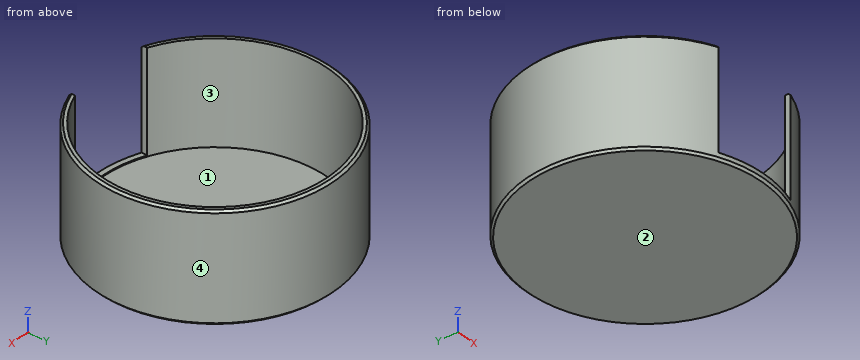
```python
from build123d import *

# Parameters (mm, degrees)
F0_R     = 55.5
F1_DEPTH = 50
F2_T     = -2.5
F4_DEPTH = 47
F5_SIZE  = 1


with BuildPart() as f1:
    # F0 (on Top) → F1 (new body)
    with BuildSketch(Plane.XY):
        Circle(F0_R)
    extrude(amount=F1_DEPTH)

    # F2
    f2_openings = [f1.faces().sort_by_distance(p)[0] for p in [
        (0, 0, 50),
    ]]
    offset(amount=F2_T, openings=f2_openings)

    # F3 (on face) → F4 (cut)
    with BuildSketch(Plane.XY.offset(50)):
        with BuildLine():
            ThreePointArc((19.8165141046, -51.841641262), (0, -55.5), (-19.8165141046, -51.841641262))
            Line((-19.8165141046, -51.841641262), (-19.8165141046, -57.2821125388))
            Line((-19.8165141046, -57.2821125388), (0, -57.2821125388))
            Line((0, -57.2821125388), (19.8165141046, -57.2821125388))
            Line((19.8165141046, -57.2821125388), (19.8165141046, -51.841641262))
        make_face()
        with BuildLine():
            ThreePointArc((19.8165141046, -49.1559331998), (0, -53), (-19.8165141046, -49.1559331998))
            Line((-19.8165141046, -49.1559331998), (-19.8165141046, -51.841641262))
            ThreePointArc((-19.8165141046, -51.841641262), (0, -55.5), (19.8165141046, -51.841641262))
            Line((19.8165141046, -51.841641262), (19.8165141046, -49.1559331998))
        make_face()
    extrude(amount=-F4_DEPTH, mode=Mode.SUBTRACT)

    # F5
    f5_edges = [f1.edges().sort_by_distance(p)[0] for p in [
        (-55.5, 0, 0),
        (-31.467709, 45.716882, 50),
    ]]
    chamfer(f5_edges, length=F5_SIZE)


solid = f1.part
```
CAD build for the part. Positions are in the model's coordinates, mm. Face numbers are marked on the shaded views. Round coordinates to 2 decimals unless told otherwise and drop trailing zeros. Order: outer loops, then holes, each group sorted by start corner. A loop starts at its lowest first (then second) coordinate and runs counter-clockwise, first axis right, second up.
Item 1: Mould opens along Y. For the marked faces 1, 2, 3 and 4 say: pulls with the +Y half, pulls with the -Y half, needs draft (parallel to the pull), parting line crosses it, or undercut.
Item 2: Saw through at C-C on z = 6. Write the cut outline in (x, y), then the cut area to 3 significant figures.
Item 3: Probe line 1 along X through (y, z) = (0, 27); line 2 along Z through (x, y) = (-32, -2.5); line 3 along X through (y, z) = (-13, 33). List the from-to ranges inside material, lowest first.
Item 4: Pin check, flat tips, straight feed: pin 1 (3 mm diameter, centred on x = 32.5, y = -40.5, fed in from -Z); pin 2 (2 mm diameter, centred on x = 20, z = 22, fed in from -Y); pin 3 (5 mm diameter, centred on x = -6.5, y = -53, fed in from +Z); pin 4 (1.5 mm diameter, centred on x = -14, z = 16.5, fed in from +Y). Stop position of each tip, or through.
Item 5: Saw through at B-B on x = 0. Write the cut outline in (y, z).
Item 6: Saw through at A-A on y = 0. Write the cut outline in (x, z), then the cut area to 3 significant figures.
Reported:
1. face 1: undercut
1. face 2: needs draft
1. face 3: undercut
1. face 4: parting line crosses it
2. outline: (-19.82, -51.84) - (-19.82, -49.16) arc R53 cw (long way) to (19.82, -49.16) - (19.82, -51.84) arc R55.5 ccw (long way) to start
2. area: 751 mm2
3. line 1: x = -55.5 to -53, 53 to 55.5
3. line 2: z = 0 to 2.5
3. line 3: x = -53.96 to -51.38, 51.38 to 53.96
4. pin 1: stops at z = 0
4. pin 2: stops at y = -51.84
4. pin 3: stops at z = 3
4. pin 4: stops at y = 53.9
5. outline: (-55.5, 1) - (-54.5, 0) - (54.5, 0) - (55.5, 1) - (55.5, 49) - (54.5, 50) - (53, 50) - (53, 2.5) - (-53, 2.5) - (-53, 3) - (-55.5, 3) - close
6. outline: (-55.5, 1) - (-54.5, 0) - (54.5, 0) - (55.5, 1) - (55.5, 49) - (54.5, 50) - (53, 50) - (53, 2.5) - (-53, 2.5) - (-53, 50) - (-54.5, 50) - (-55.5, 49) - close
6. area: 513 mm2
